Here's how the part is built. I have some questions about the finished solid (model axes, mm). A direction names the side the tool comes from. Give positions to 0.01 mm unless a question says otherwise; leave off trailing zeros. Loops run counter-clockwise (first coordinate to the right, second up) from the corner with the lowest first, then second, coordinate; pieces in that order, holes last. Notation, with made-up numbers: (-2.75, 31) - (24.25, 31) arc R32 ccw to (24.25, 67) - close; hole circle Ø10 at (43, 43). An arc over 180 degrees is marked (long way). Return JSON: item names as keys, results as strings. Group by question number.
(1) I need wall thicknesses on probe 1 along Z at (x, y) = (-0.25, 1); probe 2 along Z at (x, y) = (0.25, 4.75); probe 3 along X at (y, z) = (0.75, 9.5). Which ranges of each line are inside material? Lowest first, please. Write a range as [from, to].
(2) If we section it at B-B (x = 0): Please give me the cut outline in (y, z) (3 decimals), then the cut area to 3 significant figures.
(3) On a 3-axis mill with a long thin cutter (end or side, diameter ignored), from which of +Z, -Z, +X, -X, +Y, -Y can I reach the whole of each face in a straight line? I mean faces 1 (the cylindrical face through (-1.08, -4.88, 1.99)), 2 (the flat face through (2, -2, 3)), 3 (the flat face through (-1, 0, 1)). Say none if no direction works.
(4) If we section it at C-C (z = 15.25): Please give me the cut outline in (x, y), then the cut area to 3 significant figures.
(5) For P1, Ø1.4, axis at y = 0.5, z = 0.5, coming from the +X side; P2, Ø6, axis at x = 3.5, z = 13, coming from the +Y side; P3, Ø1, axis at x = 1.5, z = 12, coming from the -Y side; P4, Ø6, axis at y = 3.5, z = 15.5, coming from the -X side, each with a flat end and sliding along its axis, tell me the tip position at first contact or that it passes through.
(6) If we mould it in two halves opening along X, with no side actions, what happens to faces 4 (the flat face through (2, 0, 0)), 5 (the cylindrical face through (-0.54, -2.44, 10.18)), 6 (the flat face through (1, 0, 1))? For each: released by +X, released by -X, zero draft, split by the parting line, or undercut.
(7) If we section it at A-A (y = 0): Please give me the cut outline in (x, z) (3 decimals), then the cut area to 3 significant figures.
```python
from build123d import *

# Parameters (mm, degrees)
SKETCH_1_R               = 5
EXTRUDE_1_DEPTH          = 3
SKETCH_2_R               = 2.5
EXTRUDE_2_DEPTH          = 15
FILLET_1_R               = 1
SKETCH_3_W               = 2
SKETCH_3_H               = 2.5
CUT_EXTRUDE_1_DEPTH      = 6
CUT_EXTRUDE_1_DEPTH_BACK = 6.0000001
CHAMFER_1_SIZE           = 0.445


with BuildPart() as part:
    # Эскиз1 → Бобышка-Вытянуть1 (new body)
    with BuildSketch(Plane.XY):
        Circle(SKETCH_1_R)
    extrude(amount=EXTRUDE_1_DEPTH)

    # Эскиз2 → Бобышка-Вытянуть2 (add)
    with BuildSketch(Plane.XY.offset(3)):
        Circle(SKETCH_2_R)
    extrude(amount=EXTRUDE_2_DEPTH)

    # Скругление1
    fillet_1_edges = [part.edges().sort_by_distance(p)[0] for p in [
        (-5, 0, 0),
    ]]
    fillet(fillet_1_edges, radius=FILLET_1_R)

    # Эскиз3 → Вырез-Вытянуть1 (cut, two sides)
    with BuildSketch(Plane(origin=(0, 0, 0), x_dir=(1, 0, 0), z_dir=(0, 1, 0))) as cut_extrude_1_sk:
        Rectangle(SKETCH_3_W, SKETCH_3_H)
    extrude(amount=CUT_EXTRUDE_1_DEPTH, mode=Mode.SUBTRACT)
    extrude(cut_extrude_1_sk.sketch, amount=-CUT_EXTRUDE_1_DEPTH_BACK, mode=Mode.SUBTRACT)

    # Фаска1
    chamfer_1_edges = [part.edges().sort_by_distance(p)[0] for p in [
        (-2.5, 0, 18),
    ]]
    chamfer(chamfer_1_edges, length=CHAMFER_1_SIZE)


solid = part.part
```
Values:
{
 "1": {"probe 1": "[1.25, 18]", "probe 2": "[1.25, 3]", "probe 3": "[-2.38, 2.38]"},
 "2": {"outline": "(-5, 1.25) - (5, 1.25) - (5, 3) - (2.5, 3) - (2.5, 17.555) - (2.055, 18) - (-2.055, 18) - (-2.5, 17.555) - (-2.5, 3) - (-5, 3) - close", "area": "92.3 mm2"},
 "3": {"face 1": "+Z, -Z", "face 2": "+Z", "face 3": "-Z, +Y, -Y"},
 "4": {"outline": "circle Ø5 at (0, 0)", "area": "19.6 mm2"},
 "5": {"P1": "x = 5", "P2": "y = 2.45", "P3": "y = -2.29", "P4": "x = -2.45"},
 "6": {"face 4": "zero draft", "face 5": "split by the parting line", "face 6": "undercut"},
 "7": {"outline": "(-5, 1) arc R1 ccw to (-4, 0) - (-1, 0) - (-1, 1.25) - (1, 1.25) - (1, 0) - (4, 0) arc R1 ccw to (5, 1) - (5, 3) - (2.5, 3) - (2.5, 17.555) - (2.055, 18) - (-2.055, 18) - (-2.5, 17.555) - (-2.5, 3) - (-5, 3) - close", "area": "102 mm2"}
}
